from build123d import *
from OCP.BRepFilletAPI import BRepFilletAPI_MakeChamfer

# Parameters (mm, degrees)
SKETCH1_R           = 14
SKETCH1_R_2         = 12
BOSS_EXTRUDE1_DEPTH = 2
BOSS_EXTRUDE2_DEPTH = 2
CHAMFER1_SIZE       = 2
CHAMFER1_SIZE_2     = 2.300736814
FILLET1_R           = 1
SKETCH3_R           = 4
BOSS_EXTRUDE3_DEPTH = 0.5
CHAMFER2_SIZE       = 0.2
CUT_EXTRUDE1_REACH  = 22.199
SKETCH4_R           = 0.75
CHAMFER3_SIZE       = 0.2
SKETCH5_R           = 1.25
CUT_EXTRUDE2_DEPTH  = 10


with BuildPart() as part:
    # Sketch1 → Boss-Extrude1 (new body)
    with BuildSketch(Plane.XY):
        Circle(SKETCH1_R)
        Circle(SKETCH1_R_2, mode=Mode.SUBTRACT)
    extrude(amount=BOSS_EXTRUDE1_DEPTH)

    # Sketch2 → Boss-Extrude2 (add)
    with BuildSketch(Plane.XY.offset(2)):
        with BuildLine():
            ThreePointArc((-2.75, 4.763139721), (-3.889087297, 3.889087297), (-4.763139721, 2.75))
            add(Edge.make_bspline(
                [(-4.763139721, 2.75), (-7.826418416, 5.986986658), (-7, 12.124355653)],
                knots=[0.363335237, 0.363335237, 0.363335237, 1, 1, 1], degree=2))
            ThreePointArc((-7, 12.124355653), (-9.899494937, 9.899494937), (-12.124355653, 7))
            add(Edge.make_bspline(
                [(-5.5, 0), (-9.771370498, 1.27167333), (-12.124355653, 7)],
                knots=[0.363335237, 0.363335237, 0.363335237, 1, 1, 1], degree=2))
            ThreePointArc((-5.5, 0), (-5.312592045, -1.423504748), (-4.763139721, -2.75))
            add(Edge.make_bspline(
                [(-4.763139721, -2.75), (-9.098091746, -3.78438384), (-14, 0)],
                knots=[0.363335237, 0.363335237, 0.363335237, 1, 1, 1], degree=2))
            ThreePointArc((-14, 0), (-13.522961568, -3.623466631), (-12.124355653, -7))
            add(Edge.make_bspline(
                [(-2.75, -4.763139721), (-5.986986658, -7.826418416), (-12.124355653, -7)],
                knots=[0.363335237, 0.363335237, 0.363335237, 1, 1, 1], degree=2))
            ThreePointArc((-2.75, -4.763139721), (-1.423504748, -5.312592045), (0, -5.5))
            add(Edge.make_bspline(
                [(0, -5.5), (-1.27167333, -9.771370498), (-7, -12.124355653)],
                knots=[0.363335237, 0.363335237, 0.363335237, 1, 1, 1], degree=2))
            ThreePointArc((-7, -12.124355653), (-3.623466631, -13.522961568), (0, -14))
            add(Edge.make_bspline(
                [(2.75, -4.763139721), (3.78438384, -9.098091746), (0, -14)],
                knots=[0.363335237, 0.363335237, 0.363335237, 1, 1, 1], degree=2))
            ThreePointArc((2.75, -4.763139721), (3.889087297, -3.889087297), (4.763139721, -2.75))
            add(Edge.make_bspline(
                [(4.763139721, -2.75), (7.826418416, -5.986986658), (7, -12.124355653)],
                knots=[0.363335237, 0.363335237, 0.363335237, 1, 1, 1], degree=2))
            ThreePointArc((7, -12.124355653), (9.899494937, -9.899494937), (12.124355653, -7))
            add(Edge.make_bspline(
                [(5.5, 0), (9.771370498, -1.27167333), (12.124355653, -7)],
                knots=[0.363335237, 0.363335237, 0.363335237, 1, 1, 1], degree=2))
            ThreePointArc((5.5, 0), (5.312592045, 1.423504748), (4.763139721, 2.75))
            add(Edge.make_bspline(
                [(4.763139721, 2.75), (9.098091746, 3.78438384), (14, 0)],
                knots=[0.363335237, 0.363335237, 0.363335237, 1, 1, 1], degree=2))
            ThreePointArc((14, 0), (13.522961568, 3.623466631), (12.124355653, 7))
            add(Edge.make_bspline(
                [(2.75, 4.763139721), (5.986986658, 7.826418416), (12.124355653, 7)],
                knots=[0.363335237, 0.363335237, 0.363335237, 1, 1, 1], degree=2))
            ThreePointArc((2.75, 4.763139721), (1.423504748, 5.312592045), (0, 5.5))
            add(Edge.make_bspline(
                [(0, 5.5), (1.27167333, 9.771370498), (7, 12.124355653)],
                knots=[0.363335237, 0.363335237, 0.363335237, 1, 1, 1], degree=2))
            ThreePointArc((7, 12.124355653), (3.623466631, 13.522961568), (0, 14))
            add(Edge.make_bspline(
                [(-2.75, 4.763139721), (-3.78438384, 9.098091746), (0, 14)],
                knots=[0.363335237, 0.363335237, 0.363335237, 1, 1, 1], degree=2))
        make_face()
    extrude(amount=BOSS_EXTRUDE2_DEPTH)

    # Chamfer1
    chamfer1_edges_1 = [part.edges().sort_by_distance(p)[0] for p in [
        (-9.899494937, 9.899494937, 4),
    ]]
    chamfer1_side_1 = [part.faces().sort_by_distance(p)[0] for p in [
        (-9.899494937, 9.899494937, 3.96),
    ]]
    chamfer1_edges_2 = [part.edges().sort_by_distance(p)[0] for p in [
        (-13.522961568, -3.623466631, 4),
    ]]
    chamfer1_side_2 = [part.faces().sort_by_distance(p)[0] for p in [
        (-13.522961568, -3.623466631, 3.96),
    ]]
    chamfer1_edges_3 = [part.edges().sort_by_distance(p)[0] for p in [
        (13.522961568, 3.623466631, 4),
    ]]
    chamfer1_side_3 = [part.faces().sort_by_distance(p)[0] for p in [
        (13.522961568, 3.623466631, 3.96),
    ]]
    chamfer1_edges_4 = [part.edges().sort_by_distance(p)[0] for p in [
        (3.623466631, 13.522961568, 4),
    ]]
    chamfer1_side_4 = [part.faces().sort_by_distance(p)[0] for p in [
        (3.623466631, 13.522961568, 3.96),
    ]]
    chamfer1_edges_5 = [part.edges().sort_by_distance(p)[0] for p in [
        (-3.623466631, -13.522961568, 4),
    ]]
    chamfer1_side_5 = [part.faces().sort_by_distance(p)[0] for p in [
        (-3.623466631, -13.522961568, 3.96),
    ]]
    chamfer1_edges_6 = [part.edges().sort_by_distance(p)[0] for p in [
        (9.899494937, -9.899494937, 4),
    ]]
    chamfer1_side_6 = [part.faces().sort_by_distance(p)[0] for p in [
        (9.899494937, -9.899494937, 3.96),
    ]]
    chamfer1 = BRepFilletAPI_MakeChamfer(part.part.solid().wrapped)
    for e in chamfer1_edges_1:
        chamfer1.Add(CHAMFER1_SIZE - 0.0001, CHAMFER1_SIZE_2 - 0.0001, e.wrapped, chamfer1_side_1[0].wrapped)
    for e in chamfer1_edges_2:
        chamfer1.Add(CHAMFER1_SIZE - 0.0001, CHAMFER1_SIZE_2 - 0.0001, e.wrapped, chamfer1_side_2[0].wrapped)
    for e in chamfer1_edges_3:
        chamfer1.Add(CHAMFER1_SIZE - 0.0001, CHAMFER1_SIZE_2 - 0.0001, e.wrapped, chamfer1_side_3[0].wrapped)
    for e in chamfer1_edges_4:
        chamfer1.Add(CHAMFER1_SIZE - 0.0001, CHAMFER1_SIZE_2 - 0.0001, e.wrapped, chamfer1_side_4[0].wrapped)
    for e in chamfer1_edges_5:
        chamfer1.Add(CHAMFER1_SIZE - 0.0001, CHAMFER1_SIZE_2 - 0.0001, e.wrapped, chamfer1_side_5[0].wrapped)
    for e in chamfer1_edges_6:
        chamfer1.Add(CHAMFER1_SIZE - 0.0001, CHAMFER1_SIZE_2 - 0.0001, e.wrapped, chamfer1_side_6[0].wrapped)
    add(Compound.cast(chamfer1.Shape()), mode=Mode.REPLACE)  # a hair under: the kernel refuses the full size

    # Fillet1
    fillet1_edges = [part.edges().sort_by_distance(p)[0] for p in [
        (10.785366658, 4.533317219, 4),
        (9.318651204, -7.073742906, 4),
        (-1.466715454, -11.607060125, 4),
        (-10.785366658, -4.533317219, 4),
        (-9.318651204, 7.073742906, 4),
        (1.466715454, 11.607060125, 4),
    ]]
    fillet(fillet1_edges, radius=FILLET1_R)

    # Sketch3 → Boss-Extrude3 (add)
    with BuildSketch(Plane.XY.offset(4)):
        Circle(SKETCH3_R)
    extrude(amount=BOSS_EXTRUDE3_DEPTH)

    # Chamfer2
    chamfer2_edges = [part.edges().sort_by_distance(p)[0] for p in [
        (-4, 0, 4.5),
    ]]
    chamfer(chamfer2_edges, length=CHAMFER2_SIZE)

    # Sketch4 → Cut-Extrude1 (cut, up to next)
    with BuildSketch(Plane.XY.offset(4), mode=Mode.PRIVATE) as cut_extrude1_sk1:
        with Locations((-1.375, 5.13156986)):
            Circle(SKETCH4_R)
    cut_extrude1_tool1 = extrude(cut_extrude1_sk1.sketch, amount=-CUT_EXTRUDE1_REACH, mode=Mode.PRIVATE) & part.part
    # Sketch4 → Cut-Extrude1 (cut, up to next)
    with BuildSketch(Plane.XY.offset(4), mode=Mode.PRIVATE) as cut_extrude1_sk2:
        with Locations((5.13156986, -1.375)):
            Circle(SKETCH4_R)
    cut_extrude1_tool2 = extrude(cut_extrude1_sk2.sketch, amount=-CUT_EXTRUDE1_REACH, mode=Mode.PRIVATE) & part.part
    # Sketch4 → Cut-Extrude1 (cut, up to next)
    with BuildSketch(Plane.XY.offset(4), mode=Mode.PRIVATE) as cut_extrude1_sk3:
        with Locations((-3.75656986, -3.75656986)):
            Circle(SKETCH4_R)
    cut_extrude1_tool3 = extrude(cut_extrude1_sk3.sketch, amount=-CUT_EXTRUDE1_REACH, mode=Mode.PRIVATE) & part.part
    add(cut_extrude1_tool1.solids().sort_by_distance((-1.375, 5.13157, 4))[0], mode=Mode.SUBTRACT)
    add(cut_extrude1_tool2.solids().sort_by_distance((5.13157, -1.375, 4))[0], mode=Mode.SUBTRACT)
    add(cut_extrude1_tool3.solids().sort_by_distance((-3.75657, -3.75657, 4))[0], mode=Mode.SUBTRACT)

    # Chamfer3
    chamfer3_edges = [part.edges().sort_by_distance(p)[0] for p in [
        (-2.125, 5.13156986, 4),
        (4.38156986, -1.375, 4),
        (-4.50656986, -3.75656986, 4),
    ]]
    chamfer(chamfer3_edges, length=CHAMFER3_SIZE)

    # Sketch5 → Cut-Extrude2 (cut)
    with BuildSketch(Plane.XY.offset(4.5)):
        Circle(SKETCH5_R)
    extrude(amount=-CUT_EXTRUDE2_DEPTH, mode=Mode.SUBTRACT)


solid = part.part
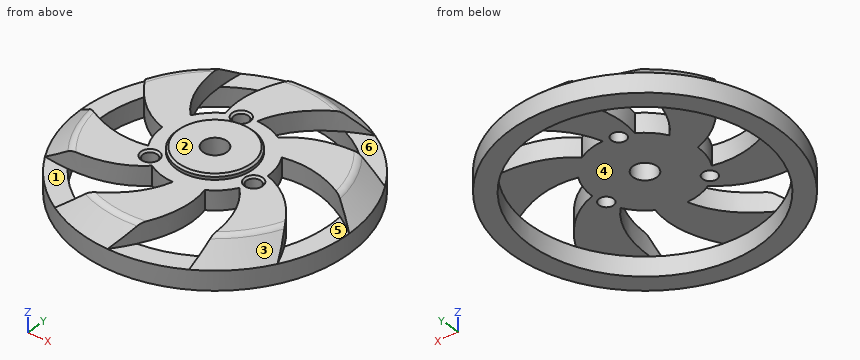
Geometry: final body of the model. Coordinates: model frame, mm. Face numbers are marked on the shaded views. A direction names the side the tool comes from. Give positions to 0.01 mm unless a question says otherwise; leave off trailing zeros. Write each loop counter-clockwise with the first axis right and the second up, starting at its lowest first coordinate (ties: lowest second). Pieces come first, ordered by that corner, then holes. Notation, with made-up numbers: (-26, 20) - (13, 20) arc R28 ccw to (13, 47) - close; hole circle Ø2 at (-19.5, 24). An arc over 180 degrees is marked (long way). Return JSON: item names as keys, results as strings. Group by question number.
1) Section B-B on x = 6.5. State how many separate pieces and enclosed holes the cut face has, plus the area to 3 significant figures.
2) Mould query, pull axis Y, two halves, no side actions, for the marked faces 1, 2 and 3. Classes: released by +Y, released by -Y, zero draft, split by the parting line, or undercut.
3) Line query: line 1 (Y direction, x = 0, z = 1.45); line 2 (X direction, y = -4.25, z = 2.4); line 3 (Z direction, x = 6, y = -0.75). Output: solid intervals per line, ascending.
4) First-contact query: P1, Ø10, axis at x = 2, y = 2, coming from the -Z side; P2, Ø5, axis at x = 2.5, y = -12, coming from the +Z side; P3, Ø0.9, axis at x = 13, y = -3.5, coming from the +Z side. Flat tips, straight axial feed; report the tip coordinate or a pass-through.
5) Set-up query: the marked faces 4, 5 and 6. Return all of +Z, -Z, +X, -X, +Y, -Y with unobstructed straight access to the full face (end or side cutting, diameter ignored); none if empty.
6) Section A-A on z = 0.7. Return the cut outline in (x, y).
Filled in:
{
 "1": {"separate pieces": "4", "enclosed holes": "0", "area": "27.4 mm^2"},
 "2": {"face 1": "undercut", "face 2": "zero draft", "face 3": "released by -Y"},
 "3": {"line 1": "y = -14 to -12, 12 to 14", "line 2": "x = -12.86 to -4.32, -3.19 to 3.49, 5.89 to 10.73", "line 3": "z = 2 to 4"},
 "4": {"P1": "stops at z = 2", "P2": "stops at z = 4", "P3": "stops at z = 2"},
 "5": {"face 4": "-Z", "face 5": "+Z", "face 6": "+Z, +X"},
 "6": {"outline": "circle Ø28 at (0, 0); hole circle Ø24 at (0, 0)"}
}
